Geometry check sheet. Reference: the model listing, model coordinates, mm. A direction names the side the tool comes from. Give positions to 0.01 mm unless a question says otherwise; leave off trailing zeros. Loops run counter-clockwise (first coordinate to the right, second up) from the corner with the lowest first, then second, coordinate; pieces in that order, holes last. Notation, with made-up numbers: (15.5, -34.5) - (53.5, -34.5) arc R10 ccw to (53.5, -25.5) - close; hole circle Ø4 at (55, 0.5). An arc over 180 degrees is marked (long way). Use a Markdown table: item, result. Add a question column.
1. Depth check by flat-ended pin: P1, Ø1.3, axis at x = 12, y = 21, coming from the -Z side; P2, Ø0.6, axis at y = 64, z = 31.5, coming from the +X side; P3, Ø8, axis at x = 11.5, y = 37.5, coming from the +Z side; P4, Ø2, axis at y = -3, z = 20.3, coming from the -X side. Enter the tip coordinate at first touch or a pass-through.
2. Cross-section at B-B on y = -3. Count the separate pieces of the cut face and the enclosed holes in it, and give its area (3 significant figures).
3. Draft check along Z on faces 1 (the flat face through (11.387, 49, -32)), 2 (the cylindrical face through (14.88, 50.43, 30.46)), 3 (the cylindrical face through (13.101, -2.941, 18.948)), 4 (the flat face through (17, 0, -4)). Enter one of: pulls with the +Z half, pulls with the -Z half, needs draft (parallel to the pull), parting line crosses it, or undercut.
4. Cross-section at A-A on x = -26.5. Enter the section's corners in (y, z), and give its area (3 significant figures).
5. Set-up check for faces 5 (the flat face through (13, 19, -3)), 6 (the flat face through (-44, 50, -38.103)), 7 (the flat face through (14, 96, -3)), 8 (the flat face through (12, 84, -3)): record each of +Z, -Z, +X, -X, +Y, -Y from which the full face is reachable in a straight line by a thin tool's end or side.
6. Material ranges on L1, parallel to Z at x = 16, y = 98; L2, parallel to Z at x = -30.5, y = 23; L3, parallel to Z at x = -35, y = 85.5, recorded low to high.
from build123d import *

# Parameters (mm, degrees)
BOSS_EXTRUDE1_DEPTH = 120
BOSS_EXTRUDE2_DEPTH = 120
SKETCH4_W           = 0.8
SKETCH4_H           = 47.4
BOSS_EXTRUDE3_DEPTH = 120
BOSS_EXTRUDE4_DEPTH = 6
SKETCH6_W           = 3.197214061
SKETCH6_H           = 10
SKETCH6_W_2         = 2.544721395
CUT_EXTRUDE1_DEPTH  = 90
SKETCH7_W           = 18.489641695
SKETCH7_H           = 120.194280457
CUT_EXTRUDE2_DEPTH  = 140
SKETCH9_W           = 8
SKETCH9_H           = 33.33003075
CUT_EXTRUDE3_DEPTH  = 4
SKETCH10_R          = 1.35
CUT_EXTRUDE4_DEPTH  = 11
SKETCH11_R          = 1.35
CUT_EXTRUDE5_DEPTH  = 11
SKETCH12_W          = 29
SKETCH12_H          = 3.5
CUT_EXTRUDE6_DEPTH  = 10
SKETCH13_W          = 93.224255338
SKETCH13_H          = 23.971951373
CUT_EXTRUDE7_DEPTH  = 103
SKETCH14_W          = 38.705642401
SKETCH14_H          = 10
CUT_EXTRUDE8_DEPTH  = 2.5
SKETCH15_R          = 1.35
CUT_EXTRUDE9_DEPTH  = 5
SKETCH16_R          = 1.35
CUT_EXTRUDE10_DEPTH = 88
SKETCH17_W          = 10.62518409
SKETCH17_H          = 1.204079054
SKETCH17_W_2        = 10.507821767
SKETCH17_W_3        = 9.64704318
SKETCH17_H_2        = 1.005507522
SKETCH17_W_4        = 10.576043604
SKETCH17_H_3        = 1.445279271
CUT_EXTRUDE11_DEPTH = 200


with BuildPart() as part:
    # Sketch1 → Boss-Extrude1 (new body)
    with BuildSketch(Plane(origin=(0, 0, 0), x_dir=(1, 0, 0), z_dir=(0, 1, 0))):
        with BuildLine():
            Line((-55.813088795, 29.403372847), (-55.813088795, -22.596627153))
            ThreePointArc((-55.813088795, -22.596627153), (-52.766075655, -30.195969229), (-45.313088795, -33.585257641))
            Line((-45.313088795, -33.585257641), (-45.313088795, -31.296627153))
            ThreePointArc((-45.313088795, -31.296627153), (-50.969943044, -28.953481402), (-53.313088795, -23.296627153))
            Line((-53.313088795, -23.296627153), (-53.313088795, 30.103372847))
            ThreePointArc((-53.313088795, 30.103372847), (-50.969943044, 35.760227097), (-45.313088795, 38.103372847))
            Line((-45.313088795, 38.103372847), (-45.313088795, 40.392003335))
            ThreePointArc((-45.313088795, 40.392003335), (-52.766075655, 37.002714924), (-55.813088795, 29.403372847))
        make_face()
        with BuildLine():
            Line((-45.313088795, -31.296627153), (-45.313088795, -33.585257641))
            ThreePointArc((-45.313088795, -33.585257641), (-45.063153419, -33.593784407), (-44.813088795, -33.596627153))
            Line((-44.813088795, -33.596627153), (7.186911205, -33.596627153))
            ThreePointArc((7.186911205, -33.596627153), (14.965085798, -30.374801746), (18.186911205, -22.596627153))
            Line((18.186911205, -22.596627153), (18.186911205, 29.403372847))
            ThreePointArc((18.186911205, 29.403372847), (14.965085798, 37.18154744), (7.186911205, 40.403372847))
            Line((7.186911205, 40.403372847), (-45.313088795, 40.403372847))
            Line((-45.313088795, 40.403372847), (-45.313088795, 40.392003335))
            Line((-45.313088795, 40.392003335), (-45.313088795, 38.103372847))
            Line((-45.313088795, 38.103372847), (7.686911205, 38.103372847))
            ThreePointArc((7.686911205, 38.103372847), (13.343765455, 35.760227097), (15.686911205, 30.103372847))
            Line((15.686911205, 30.103372847), (15.686911205, -23.296627153))
            ThreePointArc((15.686911205, -23.296627153), (13.343765455, -28.953481402), (7.686911205, -31.296627153))
            Line((7.686911205, -31.296627153), (-45.313088795, -31.296627153))
        make_face()
    extrude(amount=BOSS_EXTRUDE1_DEPTH)

    # Sketch3 → Boss-Extrude2 (add)
    with BuildSketch(Plane.XZ):
        Polygon((-49.013088795, 31.972735522), (-49.013088795, -37.623215713), (-53.336517426, -34.913867104), (-55.11106611, -29.984565206), (-55.11106611, -26.811210851), (-55.11106611, 25.452378342), (-53.652842224, 27.779331351), (-52.073193111, 30.226675048), align=None)
        Polygon((11.386911205, 31.972735522), (11.386911205, -38.487790626), (13.269736219, -37.809973621), (16.737085445, -32.276969537), (16.568342629, -31.170966754), (16.568342629, 24.789777041), (15.03852436, 28.997230807), align=None)
    extrude(amount=-BOSS_EXTRUDE2_DEPTH)

    # Sketch4 → Boss-Extrude3 (add)
    with BuildSketch(Plane.XZ):
        with Locations((10.986911205, -3.403372847)):
            Rectangle(SKETCH4_W, SKETCH4_H)
        with Locations((-48.613088795, -3.403372847)):
            Rectangle(SKETCH4_W, SKETCH4_H)
    extrude(amount=-BOSS_EXTRUDE3_DEPTH)

    # Sketch5 → Boss-Extrude4 (add)
    with BuildSketch(Plane.XZ):
        with BuildLine():
            ThreePointArc((-49.013088795, 30.389581403), (-52.154141346, 27.443915423), (-53.313088795, 23.296627153))
            Line((-53.313088795, 23.296627153), (-53.313088795, -30.103372847))
            ThreePointArc((-53.313088795, -30.103372847), (-52.154141346, -34.250661118), (-49.013088795, -37.196327098))
            Line((-49.013088795, -37.196327098), (-49.013088795, -27.103372847))
            Line((-49.013088795, -27.103372847), (-48.213088795, -27.103372847))
            Line((-48.213088795, -27.103372847), (-48.213088795, 20.296627153))
            Line((-48.213088795, 20.296627153), (-49.013088795, 20.296627153))
            Line((-49.013088795, 20.296627153), (-49.013088795, 30.389581403))
        make_face()
        with BuildLine():
            ThreePointArc((11.386911205, -37.196327098), (14.527963756, -34.250661118), (15.686911205, -30.103372847))
            Line((15.686911205, -30.103372847), (15.686911205, 23.296627153))
            ThreePointArc((15.686911205, 23.296627153), (14.527963756, 27.443915423), (11.386911205, 30.389581403))
            Line((11.386911205, 30.389581403), (11.386911205, 20.296627153))
            Line((11.386911205, 20.296627153), (10.586911205, 20.296627153))
            Line((10.586911205, 20.296627153), (10.586911205, -27.103372847))
            Line((10.586911205, -27.103372847), (11.386911205, -27.103372847))
            Line((11.386911205, -27.103372847), (11.386911205, -37.196327098))
        make_face()
    extrude(amount=BOSS_EXTRUDE4_DEPTH)

    # Sketch6 → Cut-Extrude1 (cut)
    with BuildSketch(Plane.XZ.offset(6)):
        with Locations((-49.114481764, 12.296627153)):
            Rectangle(SKETCH6_W, SKETCH6_H)
        with Locations((-49.440728097, -19.103372847)):
            Rectangle(SKETCH6_W_2, SKETCH6_H)
        with Locations((11.814550508, -19.103372847)):
            Rectangle(SKETCH6_W_2, SKETCH6_H)
        with Locations((11.488304175, 12.296627153)):
            Rectangle(SKETCH6_W, SKETCH6_H)
    extrude(amount=-CUT_EXTRUDE1_DEPTH, mode=Mode.SUBTRACT)

    # Sketch7 → Cut-Extrude2 (cut)
    with BuildSketch(Plane.XZ.offset(6)):
        with Locations((-54.557909643, -9.755963426)):
            Rectangle(SKETCH7_W, SKETCH7_H)
    extrude(amount=-CUT_EXTRUDE2_DEPTH, mode=Mode.SUBTRACT)

    # Sketch9 → Cut-Extrude3 (cut)
    with BuildSketch(Plane.ZY.offset(-10.586911205)):
        with Locations((-3.403372847, 2.334984625)):
            Rectangle(SKETCH9_W, SKETCH9_H)
    extrude(amount=-CUT_EXTRUDE3_DEPTH, mode=Mode.SUBTRACT)

    # Sketch10 → Cut-Extrude4 (cut)
    with BuildSketch(Plane.ZY.offset(-10.586911205)):
        with Locations((-10.753372847, -3)):
            Circle(SKETCH10_R)
        with Locations((3.946627153, -3)):
            Circle(SKETCH10_R)
    extrude(amount=-CUT_EXTRUDE4_DEPTH, mode=Mode.SUBTRACT)

    # Sketch11 → Cut-Extrude5 (cut)
    with BuildSketch(Plane.ZY.offset(-10.586911205)):
        with Locations((20.296627153, -3)):
            Circle(SKETCH11_R)
        with Locations((-27.103372847, -3)):
            Circle(SKETCH11_R)
    extrude(amount=-CUT_EXTRUDE5_DEPTH, mode=Mode.SUBTRACT)

    # Sketch12 → Cut-Extrude6 (cut)
    with BuildSketch(Plane(origin=(18.186911205, 0, 0), x_dir=(0, 0, -1), z_dir=(1, 0, 0))):
        with Locations((3.403372847, 97.75)):
            Rectangle(SKETCH12_W, SKETCH12_H)
    extrude(amount=-CUT_EXTRUDE6_DEPTH, mode=Mode.SUBTRACT)

    # Sketch13 → Cut-Extrude7 (cut)
    with BuildSketch(Plane(origin=(18.186911205, 0, 0), x_dir=(0, 0, -1), z_dir=(1, 0, 0))):
        with Locations((2.372000063, 114.285975687)):
            Rectangle(SKETCH13_W, SKETCH13_H)
    extrude(amount=-CUT_EXTRUDE7_DEPTH, mode=Mode.SUBTRACT)

    # Sketch14 → Cut-Extrude8 (cut)
    with BuildSketch(Plane.ZY.offset(-10.586911205)):
        with Locations((-2.056194048, 79)):
            Rectangle(SKETCH14_W, SKETCH14_H)
    extrude(amount=-CUT_EXTRUDE8_DEPTH, mode=Mode.SUBTRACT)

    # Sketch15 → Cut-Extrude9 (cut)
    with BuildSketch(Plane(origin=(18.186911205, 0, 0), x_dir=(0, 0, -1), z_dir=(1, 0, 0))):
        with Locations((23.403372847, 98.3)):
            Circle(SKETCH15_R)
        with Locations((-16.596627153, 98.3)):
            Circle(SKETCH15_R)
    extrude(amount=-CUT_EXTRUDE9_DEPTH, mode=Mode.SUBTRACT)

    # Sketch16 → Cut-Extrude10 (cut)
    with BuildSketch(Plane.XY.offset(33.596627153)):
        with Locations((-19.313088795, 98.3)):
            Circle(SKETCH16_R)
    extrude(amount=-CUT_EXTRUDE10_DEPTH, mode=Mode.SUBTRACT)

    # Sketch17 → Cut-Extrude11 (cut)
    with BuildSketch(Plane(origin=(0, 102.3, 0), x_dir=(1, 0, 0), z_dir=(0, 1, 0))):
        with Locations((-36.645164777, 38.20133332)):
            Rectangle(SKETCH17_W, SKETCH17_H)
        with Locations((1.096553781, 38.20133332)):
            Rectangle(SKETCH17_W_2, SKETCH17_H)
        with Locations((-38.338294946, -31.493873392)):
            Rectangle(SKETCH17_W_3, SKETCH17_H_2)
        with Locations((-0.803500168, -31.273987518)):
            Rectangle(SKETCH17_W_4, SKETCH17_H_3)
    extrude(amount=-CUT_EXTRUDE11_DEPTH, mode=Mode.SUBTRACT)


solid = part.part
Values found:
| question | item | result |
|---|---|---|
| 1 | P1 | stops at z = -39.59 |
| 1 | P2 | stops at x = 14.04 |
| 1 | P3 | stops at z = 33.59 |
| 1 | P4 | passes through |
| 2 | separate pieces | 5 |
| 2 | enclosed holes | 0 |
| 2 | area | 176 mm2 |
| 3 | face 1 | undercut |
| 3 | face 2 | pulls with the +Z half |
| 3 | face 3 | undercut |
| 3 | face 4 | needs draft |
| 4 | outline | (0, -40.4) - (102.3, -40.4) - (102.3, -38.1) - (0, -38.1) - close; (0, 31.3) - (102.3, 31.3) - (102.3, 33.6) - (0, 33.6) - close |
| 4 | area | 471 mm2 |
| 5 | face 5 | -X, -Y |
| 5 | face 6 | -X, +Y, -Y |
| 5 | face 7 | +X, -X |
| 5 | face 8 | -X |
| 6 | L1 | z = -35.99 to -24.72, -22.09 to -17.9, 11.1 to 15.28, 17.91 to 29.18 |
| 6 | L2 | z = -40.4 to -38.1, 31.3 to 33.6 |
| 6 | L3 | z = -40.4 to -38.8, 32 to 33.6 |
